Read the model definition and answer for the solid it produces. Units are mm, in the model's axes. Give positions to 0.01 mm unless a question says otherwise; leave off trailing zeros. Write each loop counter-clockwise with the first axis right and the second up, starting at its lowest first coordinate (ties: lowest second). Pieces come first, ordered by that corner, then holes. Notation, with made-up numbers: (-4.75, 68.25) -> (15.25, 68.25) arc R17 cw to (15.25, 82.25) -> close; hole circle Ø10 at (-39.5, 6.5). An arc over 180 degrees is marked (long way). Write item = value, one per line.
Autodesk Inventor part; units mm, degrees
ref_plane "YZ Plane" through (0, 0, 0) normal (1, 0, 0) x (0, 1, 0)
ref_plane "XZ Plane" through (0, 0, 0) normal (0, 1, 0) x (-1, 0, 0)
ref_plane "XY Plane" through (0, 0, 0) normal (0, 0, 1) x (1, 0, 0)
sketch "Skizze1" plane through (0, 0, 0) normal (0, 0, 1) x (1, 0, 0)
  circle A0 centre (13.0004, 19) radius 2.5
  arc A1 (45.6946, 0) -> (10.6946, 35) centre (10.6946, 0) ccw
  line L0 (-4, 35) -> (10.6946, 35)
  line L1 (-4, 0) -> (-4, 35)
  line L2 (45.6946, 0) -> (-4, 0)
  line L3 (13.0004, -80.4986) -> (13.0004, 19) construction
  line L4 (13.0004, 19) -> (-57.6019, 19) construction
  line L5 (13.0004, 19) -> (40.4873, -8.4869) construction
  line L6 (13.0004, 19) -> (51.8727, 19) construction
  line L7 (32.0004, 0) -> (5.4793, 26.5211)
  line L8 (5.4793, 26.5211) -> (9.215, 30.2568)
  line L9 (9.215, 30.2568) -> (35.7361, 3.7357)
  line L10 (35.7361, 3.7357) -> (32.0004, 0)
  circle A2 centre (13.0004, 19) radius 4.9033
  line L11 (32.0004, 0) -> (35.7361, 3.7357)
  line L12 (35.7361, 3.7357) -> (44.223, -4.7511)
  line L13 (44.223, -4.7511) -> (40.4873, -8.4869)
  line L14 (40.4873, -8.4869) -> (32.0004, 0)
  point P0 (0, 0)
  dimension "d0" = 45
extrude "Extrusion1" add sketch "Skizze1" along normal blind 45 contours A0 L7 | A0 L7 A2 | L7 A0 | A0 L7 A2 | L7 L8 L9 L10 A2 | L10 L12 L2 | L2 L12 L13 L14
sketch "Skizze2" plane through (0, 0, 45) normal (0, 0, 1) x (1, 0, 0)
  circle A0 centre (13.0004, 19) radius 2.5
  point P0 (0, 0)
extrude "Extrusion2" cut sketch "Skizze2" against normal through all
sketch "Skizze3" plane through (9.215, 30.2568, 0) normal (0.7071, 0.7071, 0) x (-0.7071, 0.7071, 0)
  point P0 (-14.8788, 0)
sketch "Skizze4" plane through (9.215, 30.2568, 0) normal (0.7071, 0.7071, 0) x (-0.7071, 0.7071, 0)
  line L0 (-49.5087, 0) -> (0, 0)
  line L1 (0, 0) -> (0, 45)
  line L2 (-49.5087, 45) -> (0, 45)
  line L3 (-49.5087, 0) -> (-49.5087, 45)
  line L4 (-3.2544, 2.717) -> (-46.2544, 2.717)
  line L5 (-46.2544, 2.717) -> (-46.2544, 40.717)
  line L6 (-46.2544, 40.717) -> (-3.2544, 40.717)
  line L7 (-3.2544, 40.717) -> (-3.2544, 2.717)
  line L8 (-3.2544, 2.717) -> (-46.2544, 40.717) construction
  line L9 (-46.2544, 2.717) -> (-3.2544, 40.717) construction
  point P0 (-14.8788, 0)
  point P1 (-24.7544, 21.717)
  dimension "d5" = 43
  dimension "d6" = 38
extrude "Extrusion3" cut sketch "Skizze4" against normal blind 12 contours L4 L5 L6 L7
sketch "Skizze6" plane through (5.4793, 26.5211, 0) normal (-0.7071, 0.7071, 0) x (-0.7071, -0.7071, 0)
  line L0 (-5.2831, 0) -> (0, 0)
  line L1 (0, 0) -> (0, 45)
  line L2 (-5.2831, 45) -> (0, 45)
  line L3 (-5.2831, 0) -> (-5.2831, 45)
  line L4 (-4.1416, 1.5) -> (-1.1416, 1.5)
  line L5 (-1.1416, 1.5) -> (-1.1416, 43.5)
  line L6 (-1.1416, 43.5) -> (-4.1416, 43.5)
  line L7 (-4.1416, 43.5) -> (-4.1416, 1.5)
  line L8 (-4.1416, 1.5) -> (-1.1416, 43.5) construction
  line L9 (-1.1416, 1.5) -> (-4.1416, 43.5) construction
  point P0 (22.6277, 0)
  point P1 (-2.6416, 22.5)
  dimension "d11" = 3
  dimension "d12" = 42
extrude "Extrusion5" cut sketch "Skizze6" against normal up to surface (46.2544 mm away) contours L7 L6 L5 L4
properties part number "17_Spiegelhalterung"
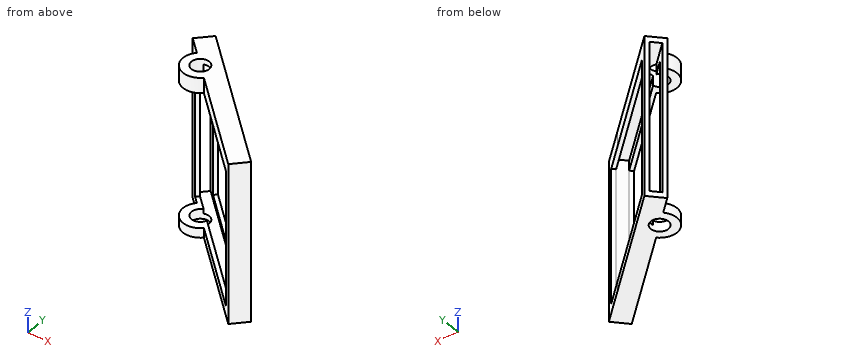
(1) Consider L1, parallel to Z at x = 10.5, y = 17; L2, parallel to Z at x = 29.5, y = 7.5; L3, parallel to X at y = 19, z = 43.9. Determine where each line is inside the solid, lowest interval first.
Checks:
L1 = 0 to 2.72, 40.72 to 45
L2 = 0 to 1.5, 43.5 to 45
L3 = 8.1 to 10.5, 15.5 to 20.47
(2) Given P1, Ø6, axis at x = 32, z = 6, coming from the +Y side; P2, Ø10, axis at x = 14.5, z = 35, coming from the -Y side; P3, Ø4, axis at y = 0, z = 39, coming from the +X side, each flat-ended and moving along its own axis, determine where each tip first touches the part or whether it passes through.
Checks:
P1 = through
P2 = 27.15
P3 = 40.5
(3) The part is cut by section C-C on y = -0.5. Determine the outline of the cut face in (x, z), plus the area to 3 significant figures.
Checks:
outline = (32.5, 0) -> (39.97, 0) -> (39.97, 2.72) -> (38.36, 2.72) -> (38.36, 1.5) -> (34.11, 1.5) -> (34.11, 2.72) -> (32.5, 2.72) -> close; (32.5, 40.72) -> (34.11, 40.72) -> (34.11, 43.5) -> (38.36, 43.5) -> (38.36, 40.72) -> (39.97, 40.72) -> (39.97, 45) -> (32.5, 45) -> close
area = 35.3 mm²
(4) The part is cut by section B-B on x = 30. Determine the outline of the cut face in (y, z).
Checks:
outline = (2, 0) -> (9.47, 0) -> (9.47, 2.72) -> (7.86, 2.72) -> (7.86, 1.5) -> (3.61, 1.5) -> (3.61, 2.72) -> (2, 2.72) -> close; (2, 40.72) -> (3.61, 40.72) -> (3.61, 43.5) -> (7.86, 43.5) -> (7.86, 40.72) -> (9.47, 40.72) -> (9.47, 45) -> (2, 45) -> close
(5) The part is cut by section D-D on y = 19. Determine the outline of the cut face in (x, z), plus the area to 3 significant figures.
Checks:
outline = (8.1, 0) -> (10.5, 0) -> (10.5, 2.72) -> (8.1, 2.72) -> close; (8.1, 40.72) -> (10.5, 40.72) -> (10.5, 45) -> (8.1, 45) -> close; (15.5, 0) -> (20.47, 0) -> (20.47, 2.72) -> (18.86, 2.72) -> (18.86, 1.5) -> (15.5, 1.5) -> close; (15.5, 43.5) -> (18.86, 43.5) -> (18.86, 40.72) -> (20.47, 40.72) -> (20.47, 45) -> (15.5, 45) -> close
area = 38.2 mm²
(6) The part is cut by section A-A on z = 26.5. Count the separate pieces of the cut face and the enclosed holes in it, plus the area to 3 significant figures.
Checks:
separate_pieces = 3
enclosed_holes = 0
area = 24.6 mm²
